Geometry: final body of the model. Coordinates: model frame, mm. Face numbers are marked on the shaded views. Round coordinates to 2 decimals unless told otherwise and drop trailing zeros. Loops run counter-clockwise (first coordinate to the right, second up) from the corner with the lowest first, then second, coordinate; pieces in that order, holes last. Notation, with made-up numbers: (17.25, 21) -> (54.25, 21) arc R9 cw to (54.25, 30) -> close; hole circle Ø9 at (46.25, 14). An arc over 180 degrees is marked (long way). Answer in a Markdown table with one row per item.
```python
from build123d import *

# Parameters (mm, degrees)
F1_DEPTH = 63.5


with BuildPart() as f1:
    # F0 (on Front) → F1 (new body, symmetric)
    with BuildSketch(Plane.XZ):
        with BuildLine():
            Line((-38.852121, 76.2), (-38.852121, 0))
            Line((-38.852121, 0), (-5.832121, 0))
            ThreePointArc((-5.832121, 0), (-3.292121, 2.54), (-5.832121, 5.08))
            Line((-5.832121, 5.08), (-31.274684, 9.333155))
            ThreePointArc((-31.274684, 9.333155), (-33.127235, 10.056062), (-34.534121, 11.461485))
            Line((-34.534121, 11.461485), (-34.534121, 63.479383))
            ThreePointArc((-34.534121, 63.479383), (-34.072711, 65.544346), (-32.776249, 67.216516))
            Line((-32.776249, 67.216516), (-11.493637, 71.207009))
            ThreePointArc((-11.493637, 71.207009), (-9.465235, 74.171598), (-12.429824, 76.2))
            Line((-12.429824, 76.2), (-38.852121, 76.2))
        make_face()
    extrude(amount=F1_DEPTH, both=True)


solid = f1.part
```
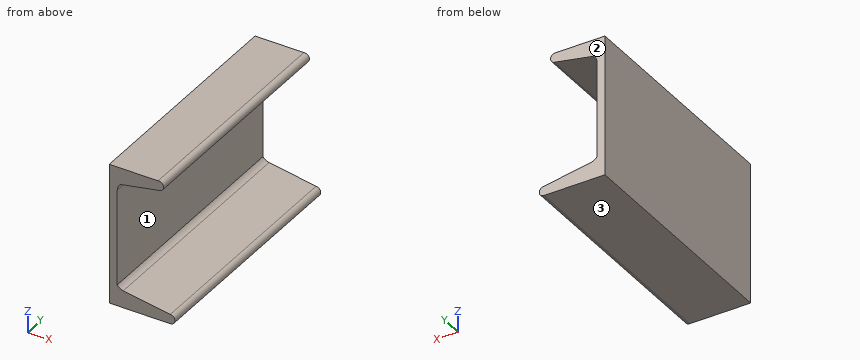
Item 1: Section query B-B, the plane z = 26.5. Output: boundary loops of the cut face in (x, y), and give its area (3 significant figures).
Ans:
| item | result |
|---|---|
| outline | (-38.85, -63.5) -> (-34.53, -63.5) -> (-34.53, 63.5) -> (-38.85, 63.5) -> close |
| area | 548 mm2 |
Item 2: First-contact query: P1, Ø1.5, axis at x = -9, y = 46, coming from the +Z side; P2, Ø2, axis at x = -9, y = -32.5, coming from the +Z side; P3, Ø12, axis at y = 22, z = 28, coming from the +X side. Flat tips, straight axial feed; report the tip coordinate or a pass-through.
Ans:
| item | result |
|---|---|
| P1 | z = 74.95 |
| P2 | z = 75.32 |
| P3 | x = -34.53 |
Item 3: Ray query, L1, parallel to X at y = -24.5, z = 40; L2, parallel to Z at x = -32, y = 40; L3, parallel to Z at x = -27, y = -20.5. Return the intervals inside material, ascending.
Ans:
| item | result |
|---|---|
| L1 | -38.85 to -34.53 |
| L2 | 0 to 9.51, 67.36 to 76.2 |
| L3 | 0 to 8.62, 68.3 to 76.2 |
Item 4: Section query A-A, the plane y = 32. Output: boundary loops of the cut face in (x, z).
Ans:
| item | result |
|---|---|
| outline | (-38.85, 0) -> (-5.83, 0) arc R2.54 ccw to (-5.83, 5.08) -> (-31.27, 9.33) arc R4.85 cw to (-34.53, 11.46) -> (-34.53, 63.48) arc R4.85 cw to (-32.78, 67.22) -> (-11.49, 71.21) arc R2.54 ccw to (-12.43, 76.2) -> (-38.85, 76.2) -> close |
Item 5: Section query C-C, the plane z = 68.5. Output: boundary loops of the cut face in (x, y), and give its area (3 significant figures).
Ans:
| item | result |
|---|---|
| outline | (-38.85, -63.5) -> (-25.93, -63.5) -> (-25.93, 63.5) -> (-38.85, 63.5) -> close |
| area | 1,640 mm2 |
Item 6: Mould query, pull axis Z, two halves, no side actions, for the marked faces 1, 2 and 3. Classes: released by +Z, released by -Z, zero draft, split by the parting line, or undercut.
Ans:
| item | result |
|---|---|
| face 1 | undercut |
| face 2 | zero draft |
| face 3 | released by -Z |
